Autodesk Inventor part; units mm, degrees
ref_plane "YZ Plane" through (0, 0, 0) normal (1, 0, 0) x (0, 1, 0)
ref_plane "XZ Plane" through (0, 0, 0) normal (0, 1, 0) x (-1, 0, 0)
ref_plane "XY Plane" through (0, 0, 0) normal (0, 0, 1) x (1, 0, 0)
sketch "Sketch8" plane through (0, 0, 0) normal (0, 1, 0) x (-1, 0, 0)
  circle A0 centre (0, 0) radius 13
  dimension "d25" = 26
extrude "Extrusion8" add sketch "Sketch8" along normal blind 2
sketch "Sketch9" plane through (0, 0, 0) normal (0, -1, 0) x (1, 0, 0)
  circle A0 centre (0, 0) radius 9.5
  dimension "d28" = 19
extrude "Extrusion9" add sketch "Sketch9" along normal blind 3
sketch "Sketch10" plane through (0, -3, 0) normal (0, -1, 0) x (1, 0, 0)
  circle A0 centre (0, 0) radius 9.5
  circle A1 centre (-9.5, 0) radius 2
  line L0 (-18.2, 0) -> (18.2, 0)
  point P0 (-9.2895, -1.9889)
  point P1 (-9.2895, 1.9889)
  dimension "d31" = 4
extrude "Extrusion10" add sketch "Sketch10" against normal up to surface (3 mm away) contours A0 L0 A1 | A1 L0 A0 picked at (-10.0838, 0.5297) picked at (-10.0838, -0.5297)
pattern_circular "Circular Pattern2" count 4 over 360 about axis through (0, 0, 0) along (0, -1, 0) of "Extrusion10"
sketch "Sketch11" plane through (0, -3, 0) normal (0, -1, 0) x (1, 0, 0)
  circle A0 centre (0, 0) radius 5.5
  dimension "d41" = 11
extrude "Extrusion11" cut sketch "Sketch11" against normal up to surface (5 mm away)
properties part number "Tapa"
CAD build for the part. Positions are in the model's coordinates, mm. A direction names the side the tool comes from. Round coordinates to 2 decimals unless told otherwise and drop trailing zeros. Order: outer loops, then holes, each group sorted by start corner. A loop starts at its lowest first (then second) coordinate and runs counter-clockwise, first axis right, second up. Notation, with made-up numbers: M 36.25,38.25 L 54.25,38.25 A6 cw 54.25,44.25 Z; hole C 9,52 d4. An arc over 180 degrees is marked long. Use one line per item in the form item = value.
Q1. Saw through at D-D on x = 8.25. Give the cut face in (y, z).
Recorded:
outline = M -3,-4.71 L 0,-4.71 L 0,-10.05 L 2,-10.05 L 2,10.05 L 0,10.05 L 0,4.71 L -3,4.71 Z
Q2. Saw through at B-B on z = 0. Give the cut face in (x, y).
Recorded:
outline = M -13,0 L -11.5,0 L -11.5,-3 L -5.5,-3 L -5.5,2 L -13,2 Z; M 5.5,-3 L 11.5,-3 L 11.5,0 L 13,0 L 13,2 L 5.5,2 Z
Q3. Which spindle directions (+Z, -Z, +X, -X, +Y, -Y) get a long thin tool onto all of the face, cutting with end or side? Do faces 1 (the flat face through (4, 0, 9)), 2 (the cylindrical face through (10.316, 0.986, 7.91)). Say none if no direction does.
Recorded:
face_1 = -Y
face_2 = +Y, -Y
Q4. Saw through at C-C on y = -2.45. Give the cut face in (x, z).
Recorded:
outline = M -9.29,-1.99 A9.5 ccw -1.99,-9.29 A2 ccw long 1.99,-9.29 A9.5 ccw 9.29,-1.99 A2 ccw long 9.29,1.99 A9.5 ccw 1.99,9.29 A2 ccw long -1.99,9.29 A9.5 ccw -9.29,1.99 A2 ccw long Z; hole C 0,0 d11
Q5. Saw through at A-A on x = 0. Give the cut face in (y, z), then the cut area to 3 significant figures.
Recorded:
outline = M -3,-11.5 L 0,-11.5 L 0,-13 L 2,-13 L 2,-5.5 L -3,-5.5 Z; M -3,5.5 L 2,5.5 L 2,13 L 0,13 L 0,11.5 L -3,11.5 Z
area = 66.0 mm^2
Q6. Probe L1, parallel to Z at x = 0, y = -1.3; L2, parallel to Z at x = 0, y = 0.95; L3, parallel to X at y = -1.85, z = 9.75. List the from-to ranges inside material, lowest first.
Recorded:
L1 = -11.5 to -5.5, 5.5 to 11.5
L2 = -13 to -5.5, 5.5 to 13
L3 = -1.98 to 1.98
Q7. Flat gauge pins, fed straight in: P1, Ø1.5, axis at x = 6.5, y = -1.5, coming from the +Z side; P2, Ø1.5, axis at y = -1, z = -8.5, coming from the -X side; P3, Ø14.5, axis at x = 0, z = 0, coming from the -Y side; P4, Ø1.5, axis at x = 5.5, y = -0.5, coming from the -Z side. Where does each tip first touch, or does it go through?
Recorded:
P1 = 7.56
P2 = -5.49
P3 = -3
P4 = -12.02
Q8. Two-plate mould, pull along X, no slides. Class faces 3 (the cylindrical face through (0, -1.5, -11.5)), 4 (the cylindrical face through (-1.19, -0.54, -5.37)), 5 (the flat face through (-6, 2, 0)): +X half, -X half, draft (parallel to the pull), parting line (faces both ways), or undercut.
Recorded:
face_3 = parting line
face_4 = undercut
face_5 = draft
